Source: three-view drawing plus pictorial views. Frame: mm from the lowest corner of the part. Give positions to 0.01 mm unless a question says otherwise; leave off trailing zeros. Order: outer loops, then holes, each group sorted by start corner. A loop starts at its lowest first (then second) coordinate and runs counter-clockwise, first axis right, second up.
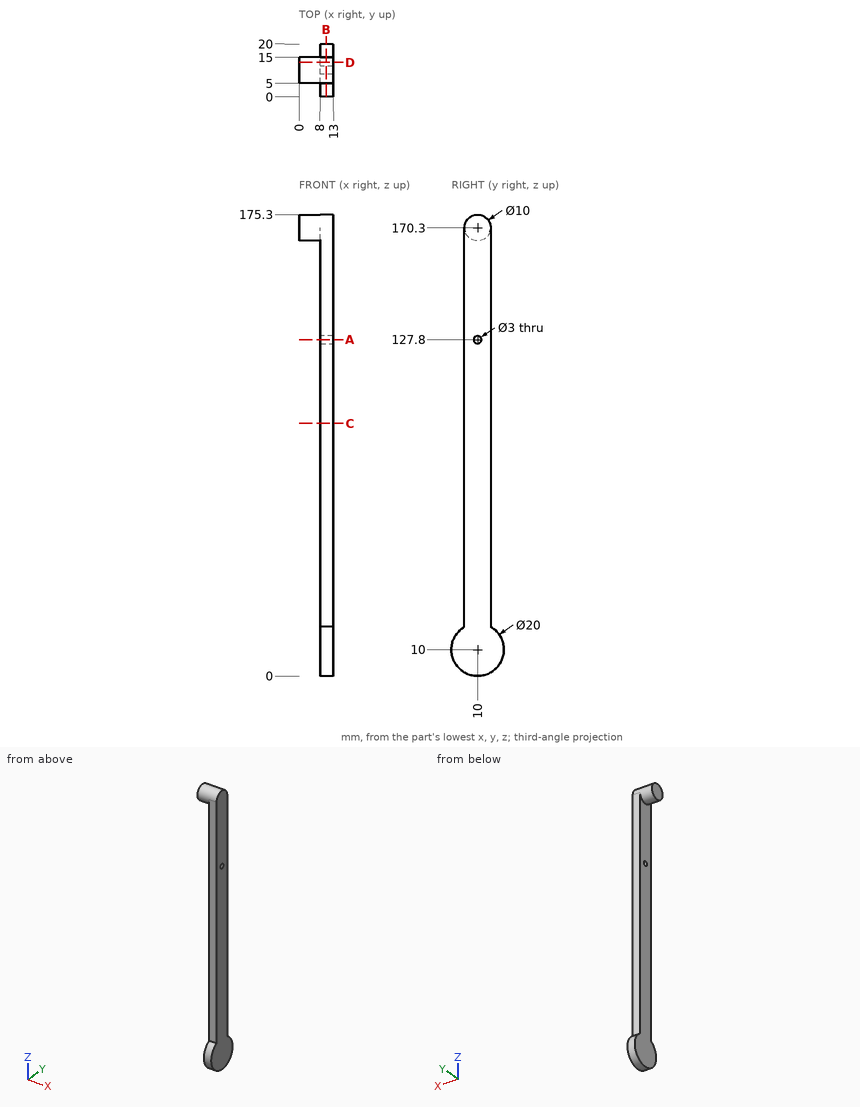
1) Section query B-B on x = 10.25. Output: boundary loops of the cut face in (y, z).
Checks:
outline: (5, 18.66) arc R10 ccw (long way) to (15, 18.66) - (15, 170.3) arc R5 ccw to (5, 170.3) - close; hole circle Ø3 at (10, 127.8)
2) Ray query, L1, parallel to Z at x = 11.75, y = 10.5; L2, parallel to X at y = 7.75, z = 127; L3, parallel to Y at x = 11.7, z = 127.8. Return the intervals inside material, ascending.
Checks:
L1: z = 0.01 to 126.39, 129.21 to 175.27
L2: x = 8 to 13
L3: y = 5 to 8.5, 11.5 to 15
3) Section query D-D on y = 13. Output: boundary loops of the cut face in (x, z), and give its area (3 significant figures).
Checks:
outline: (0, 166.3) - (8, 166.3) - (8, 0.46) - (13, 0.46) - (13, 174.3) - (0, 174.3) - close
area: 933 mm2
4) Section query C-C on z = 96. Output: boundary loops of the cut face in (x, y), and give its area (3 significant figures).
Checks:
outline: (8, 5) - (13, 5) - (13, 15) - (8, 15) - close
area: 50.0 mm2
5) Section query A-A on z = 127.8. Output: boundary loops of the cut face in (x, y), and give its area (3 significant figures).
Checks:
outline: (8, 5) - (13, 5) - (13, 8.5) - (8, 8.5) - close; (8, 11.5) - (13, 11.5) - (13, 15) - (8, 15) - close
area: 35.0 mm2
6) First-contact query: pin 1 Ø6 at (x, y) = (4, 14) entering from -Z; pin 2 Ø5.5 at (x, z) = (10, 124.5) entering from +Y; pin 3 Ø1.5 at (x, z) = (10, 57) entering from -Y. Flat tips, straight axial feed; report the tip coordinate or a pass-through.
Checks:
pin 1: stops at z = 165.4
pin 2: stops at y = 15
pin 3: stops at y = 5
